Print and shaded views of the part. All mm, measured from the part's lowest x, y and z. A direction names the side the tool comes from. Round coordinates to 2 decimals unless told otherwise and drop trailing zeros. Write each loop counter-clockwise with the first axis right and the second up, starting at its lowest first coordinate (ties: lowest second). Pieces come first, ordered by that corner, then holes. Notation, with made-up numbers: (51, 41.25) - (73, 41.25) arc R11 cw to (73, 57.25) - close; hole circle Ø7 at (-19.75, 6). An arc over 180 degrees is marked (long way). Answer as a JSON object with one key per item and string values. Group by question number.
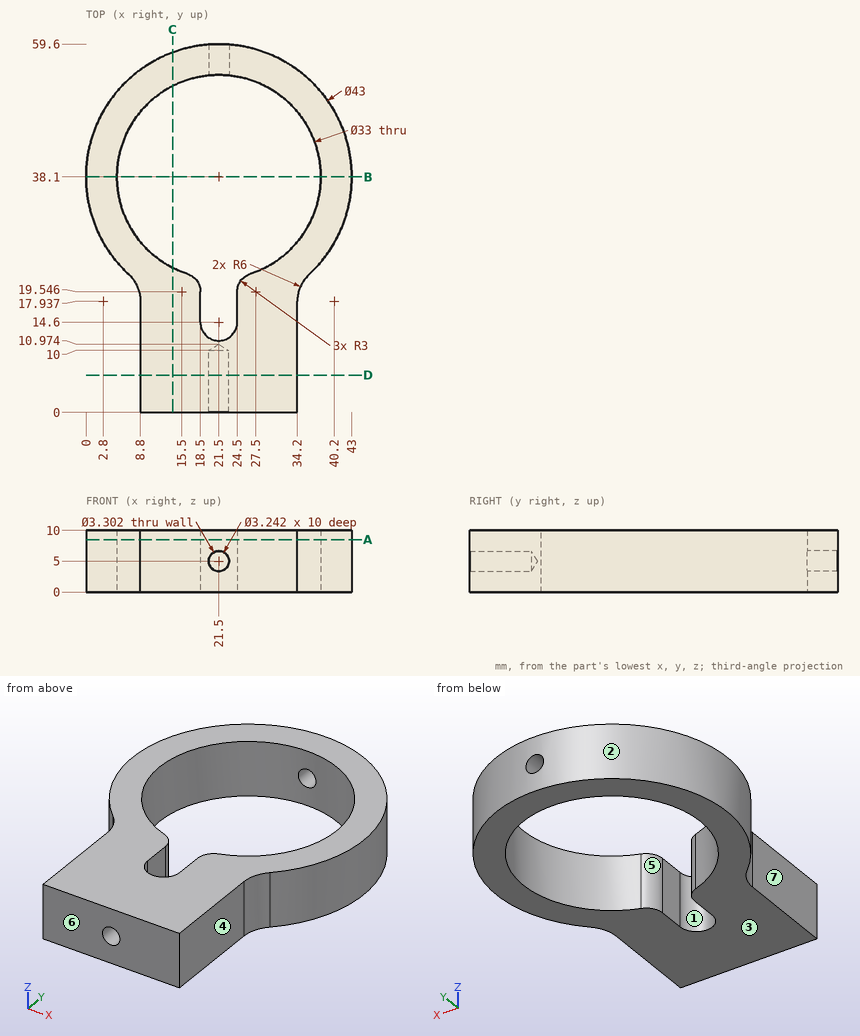
(1) Drill centre lines: line 1 (X direction, y = 38.1, z = 4.75); line 2 (X direction, y = 3, z = 5); line 3 (Y direction, x = 18, z = 1.5) (1 decimal). Where is each one in solid material? Low to high. Write a range as from..to.
(2) Slice it at D-D (y = 6). Write the cut outline in (x, z).
(3) Slice it at C-C (x = 14). Write the cut outline in (y, z).
(4) 3-axis set-ups, long thin cutter, end or side, ignore diameter. For the marked faces 4, 5, 6 and 7: which of +Z, -Z, +X, -X, +Y, -Y reach the whole face in a straight line?
(5) Pull direction X, two halves, no side cores. Call the marked faces 1, 2 and 3: pulls with the +X half, pulls with the -X half, needs draft (parallel to the pull), parting line crosses it, or undercut.
(6) Slice it at B-B (y = 38.1). Write the cut outline in (x, z), then the cut area to 4 significant figures.
(7) Slice it at A-A (z = 8.5). Write the cut outline in (x, y).
(8) Flat gauge pins, fed straight in: pin 1 (4 mm diameter, centred on y = 17.5, z = 7, fed in from +X); pin 2 (4 mm diameter, centred on y = 16.5, z = 4, fed in from -X); pin 3 (8 mm diameter, centred on x = 16.5, y = 53, fed in from +Z); pin 4 (3 mm diameter, centred on y = 7.5, z = 4.5, fed in from +X). Where does each tip first touch, or does it go through?
Answer:
{
 "1": {"line 1": "0..5, 38..43", "line 2": "8.8..19.88, 23.12..34.2", "line 3": "0..21.2, 54.2..59.3"},
 "2": {"outline": "(8.8, 0) - (34.2, 0) - (34.2, 10) - (8.8, 10) - close; hole circle Ø3.24 at (21.5, 5)"},
 "3": {"outline": "(0, 0) - (23.4, 0) - (23.4, 10) - (0, 10) - close; (52.8, 0) - (58.25, 0) - (58.25, 10) - (52.8, 10) - close"},
 "4": {"face 4": "+Z, -Z, +X, -Y", "face 5": "+Z, -Z", "face 6": "+Z, -Z, +X, -X, -Y", "face 7": "+Z, -Z, -X, -Y"},
 "5": {"face 1": "undercut", "face 2": "parting line crosses it", "face 3": "needs draft"},
 "6": {"outline": "(0, 0) - (5, 0) - (5, 10) - (0, 10) - close; (38, 0) - (43, 0) - (43, 10) - (38, 10) - close", "area": "100.0 mm²"},
 "7": {"outline": "(6.88, 22.34) arc R6 cw to (8.8, 17.94) - (8.8, 0) - (34.2, 0) - (34.2, 17.94) arc R6 cw to (36.12, 22.34) arc R21.5 ccw (long way) to start; hole (16.42, 22.4) arc R3 cw to (18.5, 19.55) - (18.5, 14.6) arc R3 ccw to (24.5, 14.6) - (24.5, 19.55) arc R3 cw to (26.58, 22.4) arc R16.5 ccw (long way) to start"},
 "8": {"pin 1": "x = 34.41", "pin 2": "x = 8.77", "pin 3": "z = 10", "pin 4": "x = 34.2"}
}
